```python
from build123d import *

# Parameters (mm, degrees)
F0_R     = 1.524
F0_W     = 23.241
F0_H     = 23.241
F0_R_2   = 8.89
F1_DEPTH = 1.5875


# Not quite as in the source:
# - a length typed as a fraction of an inch, garbled in the dataset ("3 / 203.2 mm" for 3/8 in), is restored


with BuildPart() as f1:
    # F0 (on Front) → F1 (new body, symmetric)
    with BuildSketch(Plane.XZ):
        with BuildLine():
            Line((34.925, -31.75), (40.6399987437, -31.75))
            Line((40.6399987437, -31.75), (40.6400012563, 31.75))
            ThreePointArc((40.6400012563, 31.75), (1.2563e-06, 72.3900018664), (-40.6399987437, 31.75))
            Line((-40.6399987437, 31.75), (-40.6400012563, -31.75))
            Line((-40.6400012563, -31.75), (-34.925, -31.75))
            ThreePointArc((-34.925, -31.75), (-30.4348719395, -33.6098719395), (-28.575, -38.1))
            Line((-28.575, -38.1), (-28.575, -60.706))
            Line((-28.575, -60.706), (-52.705, -60.706))
            Line((-52.705, -60.706), (-52.705, -88.9))
            Line((-52.705, -88.9), (-28.575, -88.9))
            Line((-28.575, -88.9), (-28.575, -107.95))
            ThreePointArc((-28.575, -107.95), (-24.8552561211, -116.9302561211), (-15.875, -120.65))
            Line((-15.875, -120.65), (15.875, -120.65))
            ThreePointArc((15.875, -120.65), (24.8552561211, -116.9302561211), (28.575, -107.95))
            Line((28.575, -107.95), (28.575, -88.9))
            Line((28.575, -88.9), (52.705, -88.9))
            Line((52.705, -88.9), (52.705, -60.706))
            Line((52.705, -60.706), (28.575, -60.706))
            Line((28.575, -60.706), (28.575, -38.1))
            ThreePointArc((28.575, -38.1), (30.4348719395, -33.6098719395), (34.925, -31.75))
        make_face()
        with Locations((-40.64, -86.233)):
            Circle(F0_R, mode=Mode.SUBTRACT)
        with Locations((-40.64, -63.373)):
            Circle(F0_R, mode=Mode.SUBTRACT)
        with Locations((0, -101.6)):
            Rectangle(F0_W, F0_H, mode=Mode.SUBTRACT)
        with Locations((40.64, -86.233)):
            Circle(F0_R, mode=Mode.SUBTRACT)
        with Locations((40.64, -63.373)):
            Circle(F0_R, mode=Mode.SUBTRACT)
        with Locations((0, 59.6900018664)):
            Circle(F0_R_2, mode=Mode.SUBTRACT)
    extrude(amount=F1_DEPTH, both=True)


solid = f1.part
```
Verification items for the finished model (mm, model axes). A direction names the side the tool comes from. Give positions to 0.01 mm unless a question says otherwise; leave off trailing zeros. Order: outer loops, then holes, each group sorted by start corner. A loop starts at its lowest first (then second) coordinate and runs counter-clockwise, first axis right, second up. Notation, with made-up numbers: (45, -20.5) -> (82, -20.5) arc R33 cw to (82, 17.5) -> close; hole circle Ø2 at (-3, 49). An arc over 180 degrees is marked (long way). One line per item, written item: value.
(1) Draft check along Z on faces 4 (the face through (24.756, -0.022, -117.028)), 5 (the face through (0.89, -0.02, 72.38)), 6 (the face through (-1.93, 0.02, 51.01)). Enter one of: pulls with the +Z half, pulls with the -Z half, needs draft (parallel to the pull), parting line crosses it, or undercut.
Final values:
face 4: pulls with the -Z half
face 5: pulls with the +Z half
face 6: undercut
(2) Tool access check on faces 1 (the face through (-1, -1.588, -23)), 2 (the face through (30.386, -0.022, -33.66)), 3 (the face through (-30.485, -0.022, -33.561)). Record the directions out of +Z, -Z, +X, -X, +Y, -Y that give a thin tool (end or side, any length) a straight path to the whole face; none if there is none.
Final values:
face 1: +Z, -Z, +X, -X, -Y
face 2: +X, +Y, -Y
face 3: -X, +Y, -Y
(3) Sectioned sample at B-B on y = 0.3. Count the separate pieces of the cut face and the enclosed holes in it, then the cut area to 3 significant figures.
Final values:
separate pieces: 1
enclosed holes: 6
area: 13,300 mm^2
(4) Sectioned sample at A-A on x = 0. Record the cut outline in (y, z).
Final values:
outline: (-1.59, -120.65) -> (1.59, -120.65) -> (1.59, -113.22) -> (-1.59, -113.22) -> close; (-1.59, -89.98) -> (1.59, -89.98) -> (1.59, 50.8) -> (-1.59, 50.8) -> close; (-1.59, 68.58) -> (1.59, 68.58) -> (1.59, 72.39) -> (-1.59, 72.39) -> close
(5) Sectioned sample at D-D on x = 32. Record the cut outline in (y, z), then the cut area to 3 significant figures.
Final values:
outline: (-1.59, -88.9) -> (1.59, -88.9) -> (1.59, -60.71) -> (-1.59, -60.71) -> close; (-1.59, -32.46) -> (1.59, -32.46) -> (1.59, 56.8) -> (-1.59, 56.8) -> close
area: 373 mm^2
(6) Gauge pin test, flat ends, axial feed: pin 1 (1 mm diameter, centred on y = -0.5, z = -101.5, fed in from +X) (3 decimals); pin 2 (1 mm diameter, centred on x = -36.5, y = 0, fed in from -Z); pin 3 (1 mm diameter, centred on y = -0.5, z = -44.5, fed in from -X) (3 decimals); pin 4 (2.5 mm diameter, centred on x = 40.64, z = -63.373, fed in from -Y). Record the tip position at first contact, or that the pin passes through.
Final values:
pin 1: x = 28.575
pin 2: z = -88.9
pin 3: x = -28.575
pin 4: through
(7) Sectioned sample at C-C on z = 55.5. Record the cut outline in (x, y), then the cut area to 3 significant figures.
Final values:
outline: (-32.98, -1.59) -> (-7.84, -1.59) -> (-7.84, 1.59) -> (-32.98, 1.59) -> close; (7.84, -1.59) -> (32.98, -1.59) -> (32.98, 1.59) -> (7.84, 1.59) -> close
area: 160 mm^2
(8) Scan lines: line 1 along X through (y, z) = (-0.95, -94) (1 decimal); line 2 along X through (y, z) = (0.15, 12); line 3 along Z through (x, y) = (-42.5, 0.9). Record each from-to range of solid material in increasing order. Write a range as [from, to].
Final values:
line 1: [-28.6, -11.6], [11.6, 28.6]
line 2: [-40.64, 40.64]
line 3: [-88.9, -60.71]
